```python
from build123d import *

# Parameters (mm, degrees)
CYLINDER005_R     = 3
CYLINDER005_DEPTH = 3
CYLINDER006_R     = 3
CYLINDER006_DEPTH = 3
BOX004_W          = 10
BOX004_H          = 6
BOX004_DEPTH      = 10
BOX005_W          = 10
BOX005_H          = 6
BOX005_DEPTH      = 10
CYLINDER010_R     = 1.65
CYLINDER010_DEPTH = 42
CYLINDER009_R     = 1.65
CYLINDER009_DEPTH = 42
BOX006_W          = 6
BOX006_H          = 32
BOX006_DEPTH      = 12
CYLINDER007_R     = 7
CYLINDER007_DEPTH = 6
CYLINDER008_R     = 7
CYLINDER008_DEPTH = 6
BOX001_W          = 20
BOX001_H          = 24
BOX001_DEPTH      = 17
BOX_W             = 20
BOX_H             = 15
BOX_DEPTH         = 5
BOX003_W          = 3
BOX003_H          = 39
BOX003_DEPTH      = 17
BOX007_W          = 3
BOX007_H          = 39
BOX007_DEPTH      = 17


with BuildPart() as cylinder005:
    # Cylinder005 → Cylinder005 (new body)
    with BuildSketch(Plane(origin=(6, 22, 0), x_dir=(1, 0, 0), z_dir=(0, 0, 1))):
        Circle(CYLINDER005_R)
    extrude(amount=CYLINDER005_DEPTH)


with BuildPart() as fusion001001001004:
    # Cylinder006 → Cylinder006 (new body)
    with BuildSketch(Plane(origin=(-6, 22, 0), x_dir=(1, 0, 0), z_dir=(0, 0, 1))):
        Circle(CYLINDER006_R)
    extrude(amount=CYLINDER006_DEPTH)

    # Fusion001001001004: union Cylinder005
    add(cylinder005.part)


with BuildPart() as fusion001001001004_1:
    # Fusion001001001004 placement: moved
    add(fusion001001001004.part.moved(Location((0, 0, 14))))


with BuildPart() as cube004:
    # Box004 → Box004 (new body)
    with BuildSketch(Plane(origin=(6, 19, 14), x_dir=(1, 0, 0), z_dir=(0, 0, 1))):
        with Locations((5, 3)):
            Rectangle(BOX004_W, BOX004_H)
    extrude(amount=BOX004_DEPTH)


with BuildPart() as fusion001001001005:
    # Box005 → Box005 (new body)
    with BuildSketch(Plane(origin=(-16, 19, 14), x_dir=(1, 0, 0), z_dir=(0, 0, 1))):
        with Locations((5, 3)):
            Rectangle(BOX005_W, BOX005_H)
    extrude(amount=BOX005_DEPTH)

    # Fusion001001001005: union Cube004
    add(cube004.part)


with BuildPart() as cylinder010:
    # Cylinder010 → Cylinder010 (new body)
    with BuildSketch(Plane(origin=(-6, 22, 0), x_dir=(1, 0, 0), z_dir=(0, 0, 1))):
        Circle(CYLINDER010_R)
    extrude(amount=CYLINDER010_DEPTH)


with BuildPart() as fusion001001001003:
    # Cylinder009 → Cylinder009 (new body)
    with BuildSketch(Plane(origin=(6, 22, 0), x_dir=(1, 0, 0), z_dir=(0, 0, 1))):
        Circle(CYLINDER009_R)
    extrude(amount=CYLINDER009_DEPTH)

    # Fusion001001001003: union Cylinder010
    add(cylinder010.part)


with BuildPart() as cube006:
    # Box006 → Box006 (new body)
    with BuildSketch(Plane(origin=(-3, 13, 0), x_dir=(1, 0, 0), z_dir=(0, 0, 1))):
        with Locations((3, 16)):
            Rectangle(BOX006_W, BOX006_H)
    extrude(amount=BOX006_DEPTH)


with BuildPart() as cylinder007:
    # Cylinder007 → Cylinder007 (new body)
    with BuildSketch(Plane(origin=(0, 32, 0), x_dir=(1, 0, 0), z_dir=(0, 0, 1))):
        Circle(CYLINDER007_R)
    extrude(amount=CYLINDER007_DEPTH)


with BuildPart() as fusion:
    # Cylinder008 → Cylinder008 (new body)
    with BuildSketch(Plane(origin=(0, 12, 0), x_dir=(1, 0, 0), z_dir=(0, 0, 1))):
        Circle(CYLINDER008_R)
    extrude(amount=CYLINDER008_DEPTH)

    # Fusion: union Cylinder007
    add(cylinder007.part)


with BuildPart() as cube001:
    # Box001 → Box001 (new body)
    with BuildSketch(Plane(origin=(-10, 15, 0), x_dir=(1, 0, 0), z_dir=(0, 0, 1))):
        with Locations((10, 12)):
            Rectangle(BOX001_W, BOX001_H)
    extrude(amount=BOX001_DEPTH)


with BuildPart() as cube:
    # Box → Box (new body)
    with BuildSketch(Plane(origin=(-10, 0, 12), x_dir=(1, 0, 0), z_dir=(0, 0, 1))):
        with Locations((10, 7.5)):
            Rectangle(BOX_W, BOX_H)
    extrude(amount=BOX_DEPTH)


with BuildPart() as cube003:
    # Box003 → Box003 (new body)
    with BuildSketch(Plane(origin=(-10, 0, 0), x_dir=(1, 0, 0), z_dir=(0, 0, 1))):
        with Locations((1.5, 19.5)):
            Rectangle(BOX003_W, BOX003_H)
    extrude(amount=BOX003_DEPTH)


with BuildPart() as base_endstop_mount_template:
    # Box007 → Box007 (new body)
    with BuildSketch(Plane(origin=(7, 0, 0), x_dir=(1, 0, 0), z_dir=(0, 0, 1))):
        with Locations((1.5, 19.5)):
            Rectangle(BOX007_W, BOX007_H)
    extrude(amount=BOX007_DEPTH)

    # Fusion001001001008: union Cube001, Cube, Cube003
    add(cube001.part)
    add(cube.part)
    add(cube003.part)

    # Cut002008023012009006003002002: cut Fusion
    add(fusion.part, mode=Mode.SUBTRACT)

    # Cut002008023012009006003002003: cut Cube006
    add(cube006.part, mode=Mode.SUBTRACT)

    # Cut002008023012009006003002004: cut Fusion001001001003
    add(fusion001001001003.part, mode=Mode.SUBTRACT)

    # Cut002008023012009006003002005: cut Fusion001001001005
    add(fusion001001001005.part, mode=Mode.SUBTRACT)

    # Cut002008023012009006003002006: cut Fusion001001001004
    add(fusion001001001004_1.part, mode=Mode.SUBTRACT)


solid = base_endstop_mount_template.part
```
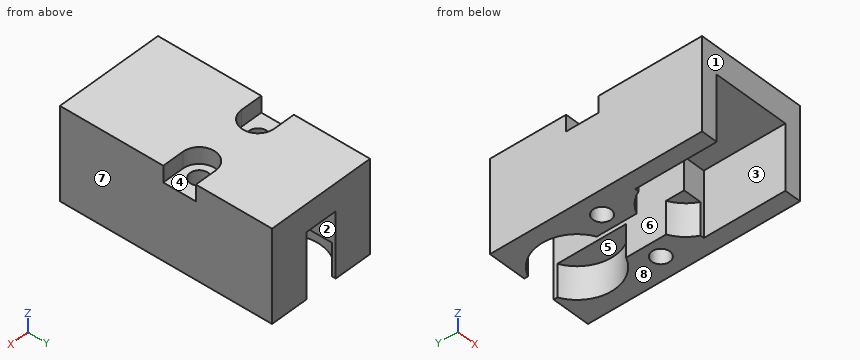
For this review, take the finished solid that the model builds, in its own axes (mm). Face numbers are marked on the shaded views. A direction names the side the tool comes from. Coordinates: 2 decimals unless noted, no trailing zeros. Order: outer loops, then holes, each group sorted by start corner. A loop starts at its lowest first (then second) coordinate and runs counter-clockwise, first axis right, second up. Notation, with made-up numbers: (46.5, 41) - (65.5, 41) arc R12 ccw to (65.5, 48) - close; hole circle Ø8 at (-4, -21). An arc over 180 degrees is marked (long way). Answer as a JSON object with one key per item and string values. Group by question number.
1. The part is to be moulded in two halves that separate along X. For the marked faces 6, 7 and 8, say which applies: pulls with the +X half, pulls with the -X half, needs draft (parallel to the pull), parting line crosses it, or undercut.
2. We need section B-B on y = 22. State the section outline as (x, z) points.
3. We need section C-C on x = -2.5. State the section outline as (y, z) points, then the cut area to 3 significant figures.
4. For the marked faces 1, 2, 3, 4 and 5, list the 3-axis set-ups (+Z, -Z, +X, -X, +Y, -Y) from which the entire face can be reached by the end or side of a thin tool; tool diameter is ignored.
5. We need section A-A on z = 4.75. State the section outline as (x, y) points, then the cut area to 3 significant figures.
6. We need section D-D on y = 8. State the section outline as (x, z) points.
7. Clearance check with flat-ended pins moving along their axes: P1, Ø1, axis at x = -1, y = 26.5, coming from the -Z side; P2, Ø3, axis at x = -4, z = 5, coming from the -Y side; P3, Ø4.5, axis at x = -6, y = 22, coming from the +Z side. State where each tip first meets the part, or that it passes through.
8. For probe 1 along X at (y, z) = (22, 11); probe 2 along X at (y, z) = (8, 9.5); probe 3 along Y at (x, z) = (-8, 15.5), list the stretches that pass through material, from the lowest coordinate up.
Final values:
{
 "1": {"face 6": "undercut", "face 7": "pulls with the +X half", "face 8": "needs draft"},
 "2": {"outline": "(-10, 0) - (-7.65, 0) - (-7.65, 14) - (-10, 14) - close; (-4.35, 0) - (-3, 0) - (-3, 12) - (3, 12) - (3, 0) - (4.35, 0) - (4.35, 14) - (3, 14) - (3, 17) - (-3, 17) - (-3, 14) - (-4.35, 14) - close; (7.65, 0) - (10, 0) - (10, 14) - (7.65, 14) - close"},
 "3": {"outline": "(0, 12) - (39, 12) - (39, 17) - (0, 17) - close", "area": "195 mm²"},
 "4": {"face 1": "+Z, -Z, +X, -X, -Y", "face 2": "-Z, +Y, -Y", "face 3": "-Z, -Y", "face 4": "+Z, +X", "face 5": "-Z"},
 "5": {"outline": "(-10, 0) - (-7, 0) - (-7, 15) - (-6.32, 15) arc R7 cw to (-3, 18.32) - (-3, 25.68) arc R7 cw to (-3, 38.32) - (-3, 39) - (-10, 39) - close; (3, 18.32) arc R7 cw to (6.32, 15) - (7, 15) - (7, 0) - (10, 0) - (10, 39) - (3, 39) - (3, 38.32) arc R7 cw to (3, 25.68) - close; hole circle Ø3.3 at (-6, 22); hole circle Ø3.3 at (6, 22)", "area": "323 mm²"},
 "6": {"outline": "(-10, 0) - (-7, 0) - (-7, 12) - (7, 12) - (7, 0) - (10, 0) - (10, 17) - (-10, 17) - close"},
 "7": {"P1": "z = 12", "P2": "y = 15", "P3": "z = 14"},
 "8": {"probe 1": "-10 to -7.65, -4.35 to -3, 3 to 4.35, 7.65 to 10", "probe 2": "-10 to -7, 7 to 10", "probe 3": "0 to 19, 25 to 39"}
}
